Build history of the part. All positions in model axes, mm. A direction names the side the tool comes from. Round coordinates to 2 decimals unless told otherwise and drop trailing zeros. Loops run counter-clockwise (first coordinate to the right, second up) from the corner with the lowest first, then second, coordinate; pieces in that order, holes last. Notation, with made-up numbers: (80, 77.25) -> (106, 77.25) arc R15 ccw to (106, 90.25) -> close; hole circle Ø3 at (78, 52.5). An arc over 180 degrees is marked (long way). Put each result on its own line as item: value. Start each with the question number.
```python
from build123d import *

# Parameters (mm, degrees)
SKETCH1_R           = 6.35
BOSS_EXTRUDE1_DEPTH = 6.35
SKETCH2_R           = 6.35
SKETCH2_R_2         = 3.175
BOSS_EXTRUDE2_DEPTH = 6.35
CUT_EXTRUDE1_REACH  = 37.549
CUT_EXTRUDE2_REACH  = 37.549
SKETCH5_R           = 1.5875
CUT_EXTRUDE3_DEPTH  = 36.548658906
MOVE_FACE1_BY       = 0.508
MOVE_FACE2_BY       = 0.254
MOVE_FACE2_2_BY     = 0.254
MOVE_FACE2_3_BY     = 0.254
MOVE_FACE2_4_BY     = 0.254


with BuildPart() as part:
    # Sketch1 → Boss-Extrude1 (new body)
    with BuildSketch(Plane.XY):
        with BuildLine():
            Line((-2.425484171, -6.35), (27.305, -6.35))
            Line((27.305, -6.35), (27.305, 6.35))
            Line((27.305, 6.35), (-2.425484171, 6.35))
            ThreePointArc((-2.425484171, 6.35), (-9.525, 9.525), (-16.624515829, 6.35))
            Line((-16.624515829, 6.35), (-27.305, 6.35))
            Line((-27.305, 6.35), (-27.305, -6.35))
            Line((-27.305, -6.35), (-16.624515829, -6.35))
            ThreePointArc((-16.624515829, -6.35), (-9.525, -9.525), (-2.425484171, -6.35))
        make_face()
        with Locations((-9.525, 0)):
            Circle(SKETCH1_R, mode=Mode.SUBTRACT)
    extrude(amount=BOSS_EXTRUDE1_DEPTH)

    # Sketch2 → Boss-Extrude2 (add)
    with BuildSketch(Plane.XY.offset(6.35)):
        with Locations((27.305, 0)):
            Circle(SKETCH2_R)
        with Locations((27.305, 0)):
            Circle(SKETCH2_R_2, mode=Mode.SUBTRACT)
    extrude(amount=-BOSS_EXTRUDE2_DEPTH)

    # Sketch3 → Cut-Extrude1 (cut, up to next)
    with BuildSketch(Plane.XY.offset(6.35), mode=Mode.PRIVATE) as cut_extrude1_sk1:
        with BuildLine():
            ThreePointArc((27.305, 3.175), (24.13, 0), (27.305, -3.175))
            Line((27.305, -3.175), (27.305, 3.175))
        make_face()
    cut_extrude1_tool1 = extrude(cut_extrude1_sk1.sketch, amount=-CUT_EXTRUDE1_REACH, mode=Mode.PRIVATE) & part.part
    add(cut_extrude1_tool1.solids().sort_by_distance((25.957488, 0, 6.35))[0], mode=Mode.SUBTRACT)

    # Sketch4 → Cut-Extrude2 (cut, up to next)
    with BuildSketch(Plane.XY.offset(6.35), mode=Mode.PRIVATE) as cut_extrude2_sk1:
        with BuildLine():
            Line((8.255, 3.175), (27.305, 3.175))
            ThreePointArc((27.305, 3.175), (30.48, 0), (27.305, -3.175))
            Line((27.305, -3.175), (8.255, -3.175))
            ThreePointArc((8.255, -3.175), (5.08, 0), (8.255, 3.175))
        make_face()
    cut_extrude2_tool1 = extrude(cut_extrude2_sk1.sketch, amount=-CUT_EXTRUDE2_REACH, mode=Mode.PRIVATE) & part.part
    add(cut_extrude2_tool1.solids().sort_by_distance((17.78, 0, 6.35))[0], mode=Mode.SUBTRACT)

    # Sketch5 → Cut-Extrude3 (cut, through all)
    with BuildSketch(Plane.XY.offset(6.35)):
        with Locations((-24.13, 3.175)):
            Circle(SKETCH5_R)
        with Locations((-24.13, -3.175)):
            Circle(SKETCH5_R)
    extrude(amount=-CUT_EXTRUDE3_DEPTH, mode=Mode.SUBTRACT)

    # Move Face1: a face moved inward by 0.508
    extrude(part.faces().sort_by_distance((0.343641582, 0, 6.35))[0], amount=MOVE_FACE1_BY, dir=(0, 0, -1), mode=Mode.SUBTRACT)

    # Move Face2: a curved face moved inward by 0.254
    add(Solid.thicken(part.faces().sort_by_distance((30.48, 0, 2.921))[0], -MOVE_FACE2_BY), mode=Mode.SUBTRACT)

    # Move Face2 2: a face moved inward by 0.254
    extrude(part.faces().sort_by_distance((17.78, 3.175, 2.921))[0], amount=MOVE_FACE2_2_BY, dir=(0, 1, 0), mode=Mode.SUBTRACT)

    # Move Face2 3: a curved face moved inward by 0.254
    add(Solid.thicken(part.faces().sort_by_distance((5.08, 0, 2.921))[0], -MOVE_FACE2_3_BY), mode=Mode.SUBTRACT)

    # Move Face2 4: a face moved inward by 0.254
    extrude(part.faces().sort_by_distance((17.78, -3.175, 2.921))[0], amount=MOVE_FACE2_4_BY, dir=(0, -1, 0), mode=Mode.SUBTRACT)


solid = part.part
```
Item 1: 3-axis set-ups, long thin cutter, end or side, ignore diameter. For faces 4 (the face through (-22, 6.35, 3)), 5 (the face through (-22, -6.35, 3)), 6 (the face through (18, -3.429, 3)), 7 (the face through (12, -6.35, 3)): which of +Z, -Z, +X, -X, +Y, -Y reach the whole face in a straight line?
Item 2: Pull direction Y, two halves, no side cores. Call faces 1 (the face through (13, 6.35, 3)), 2 (the face through (-22.664, -3.783, 2.962)), 3 (the face through (3, 0, 0)): +Y half, -Y half, draft (parallel to the pull), parting line (faces both ways), or undercut.
Item 3: Drop flat-ended pins along their axis: pin 1 (1.8 mm diameter, centred on x = 13, z = 4, fed in from +Y); pin 2 (1.8 mm diameter, centred on x = 20, z = 3.5, fed in from -Y); pin 3 (1.5 mm diameter, centred on y = -3.5, z = 1.5, fed in from +X); pin 4 (1.9 mm diameter, centred on x = -24.13, y = 3.175, fed in from -Z). Give the stop position or say it passes through.
Item 4: Cut at D-D on z = 2. State how many separate pieces and enclosed holes the cut face has, then the cut area to 3 significant figures.
Item 5: Cut at B-B on x = 20. Write the cut outline in (y, z).
Item 6: Cut at A-A on y = 0. Write the cut outline in (x, z) (3 decimals), then the cut area to 3 significant figures.
Item 7: Wall check: line 1 (Y direction, x = -24.13, z = 4.3); line 2 (Y direction, x = 11, z = 0.5); line 3 (X direction, y = -4, z = 2.45) (3 decimals). Give the ranges that are in metal, low to high. Write a range as from..to.
Item 8: Cut at C-C on x = -24.13. Write the cut outline in (y, z), then the cut area to 3 significant figures.
Ans:
1. face 4: +Z, -Z, -X, +Y
1. face 5: +Z, -Z, -X, -Y
1. face 6: +Z, -Z
1. face 7: +Z, -Z, +X, -Y
2. face 1: +Y half
2. face 2: undercut
2. face 3: draft
3. pin 1: stops at y = 6.35
3. pin 2: stops at y = -6.35
3. pin 3: stops at x = 33.03
3. pin 4: passes through
4. separate pieces: 1
4. enclosed holes: 4
4. area: 509 mm2
5. outline: (-6.35, 0) -> (-3.43, 0) -> (-3.43, 5.84) -> (-6.35, 5.84) -> close; (3.43, 0) -> (6.35, 0) -> (6.35, 5.84) -> (3.43, 5.84) -> close
6. outline: (-27.305, 0) -> (-15.875, 0) -> (-15.875, 5.842) -> (-27.305, 5.842) -> close; (-3.175, 0) -> (4.826, 0) -> (4.826, 5.842) -> (-3.175, 5.842) -> close; (30.734, 0) -> (33.655, 0) -> (33.655, 5.842) -> (30.734, 5.842) -> close
6. area: 131 mm2
7. line 1: y = -6.35..-4.76, -1.59..1.59, 4.76..6.35
7. line 2: y = -6.35..-3.43, 3.43..6.35
7. line 3: x = -27.305..-25.486, -22.774..-14.457, -4.593..32.237
8. outline: (-6.35, 0) -> (-4.76, 0) -> (-4.76, 5.84) -> (-6.35, 5.84) -> close; (-1.59, 0) -> (1.59, 0) -> (1.59, 5.84) -> (-1.59, 5.84) -> close; (4.76, 0) -> (6.35, 0) -> (6.35, 5.84) -> (4.76, 5.84) -> close
8. area: 37.1 mm2
